Verification items for the finished model (mm, model axes). A direction names the side the tool comes from. Round coordinates to 2 decimals unless told otherwise and drop trailing zeros. Order: outer loops, then holes, each group sorted by start corner. A loop starts at its lowest first (then second) coordinate and runs counter-clockwise, first axis right, second up. Notation, with made-up numbers: (4.5, 28.25) -> (44.5, 28.25) arc R17 cw to (44.5, 37.25) -> close; hole circle Ø4 at (11.25, 34). An arc over 180 degrees is marked (long way). Put each result on its own line as item: value.
from build123d import *

# Parameters (mm, degrees)
ESQUISSE1_R             = 8
BOSS_EXTRU_1_DEPTH      = 5
ESQUISSE2_W             = 30
ESQUISSE2_H             = 12
BOSS_EXTRU_2_DEPTH      = 10.5
ESQUISSE4_W             = 30
ESQUISSE4_H             = 5
BOSS_EXTRU_3_DEPTH      = 45
ENL_V_START             = -10
ESQUISSE6_R             = 8
ENL_V_MAT_EXTRU_3_DEPTH = 10
ESQUISSE8_W             = 8
ESQUISSE8_H             = 8
ESQUISSE8_R             = 2.3
BOSS_EXTRU_4_DEPTH      = 8
ENL_V_MAT_EXTRU_4_DEPTH = 2
ENL_V_MAT_EXTRU_5_DEPTH = 50
ENL_V_MAT_EXTRU_6_DEPTH = 50
BOSS_EXTRU_5_DEPTH      = 10.5
BOSS_EXTRU_7_DEPTH      = 15


with BuildPart() as part:
    # Esquisse1 → Boss.-Extru.1 (new body)
    with BuildSketch(Plane.XY):
        Polygon((0, 0), (15, 0), (15, 45), (-15, 45), (-15, 0), align=None)
        with Locations((0, 28)):
            Circle(ESQUISSE1_R, mode=Mode.SUBTRACT)
    extrude(amount=-BOSS_EXTRU_1_DEPTH)

    # Esquisse2 → Boss.-Extru.2 (add)
    with BuildSketch(Plane(origin=(0, 0, -5), x_dir=(-1, 0, 0), z_dir=(0, 0, -1))):
        with Locations((0, 6)):
            Rectangle(ESQUISSE2_W, ESQUISSE2_H)
    extrude(amount=BOSS_EXTRU_2_DEPTH)

    # Esquisse4 → Boss.-Extru.3 (add)
    with BuildSketch(Plane.XZ):
        with Locations((0, -18)):
            Rectangle(ESQUISSE4_W, ESQUISSE4_H)
    extrude(amount=-BOSS_EXTRU_3_DEPTH)

    # Esquisse6 → Enlèv. mat.-Extru.3 (cut)
    with BuildSketch(Plane(origin=(0, 0, -20.5), x_dir=(-1, 0, 0), z_dir=(0, 0, -1)).offset(ENL_V_START)):
        with Locations(Location((0, 28, 0), (0, 0, 180))):
            Circle(ESQUISSE6_R)
    extrude(amount=ENL_V_MAT_EXTRU_3_DEPTH, mode=Mode.SUBTRACT)

    # Esquisse8 → Boss.-Extru.4 (add)
    # profile 1 of 4: a face of its own
    with BuildSketch(Plane.XZ):
        with Locations((-11, 4)):
            Rectangle(ESQUISSE8_W, ESQUISSE8_H)
        with Locations(Location((-11, 4, 0), (0, 0, 270))):
            Circle(ESQUISSE8_R, mode=Mode.SUBTRACT)
    # profile 2 of 4: a face of its own
    with BuildSketch(Plane.XZ):
        with Locations((11, 4)):
            Rectangle(ESQUISSE8_W, ESQUISSE8_H)
        with Locations(Location((11, 4, 0), (0, 0, 270))):
            Circle(ESQUISSE8_R, mode=Mode.SUBTRACT)
    # profile 3 of 4: a face of its own
    with BuildSketch(Plane.XZ):
        with Locations((-11, -24.5)):
            Rectangle(ESQUISSE8_W, ESQUISSE8_H)
        with Locations(Location((-11, -24.5, 0), (0, 0, 270))):
            Circle(ESQUISSE8_R, mode=Mode.SUBTRACT)
    # profile 4 of 4: a face of its own
    with BuildSketch(Plane.XZ):
        with Locations((11, -24.5)):
            Rectangle(ESQUISSE8_W, ESQUISSE8_H)
        with Locations(Location((11, -24.5, 0), (0, 0, 270))):
            Circle(ESQUISSE8_R, mode=Mode.SUBTRACT)
    extrude(amount=-BOSS_EXTRU_4_DEPTH)

    # Esquisse9 → Enlèv. mat.-Extru.4 (cut)
    with BuildSketch(Plane.XZ):
        Polygon((-15, 8), (-15, -28.5), (-7, -28.5), (-7, -20.5), (7, -20.5), (7, -28.5), (15, -28.5), (15, 8), (7, 8), (7, 0), (-7, 0), (-7, 8), align=None)
    extrude(amount=-ENL_V_MAT_EXTRU_4_DEPTH, mode=Mode.SUBTRACT)

    # Esquisse10 → Enlèv. mat.-Extru.5 (cut)
    with BuildSketch(Plane.ZY.offset(15)):
        with BuildLine():
            Line((-13.25, 2), (-7.25, 2))
            Line((-7.25, 2), (-7.25, 5.5))
            ThreePointArc((-7.25, 5.5), (-10.25, 8.5), (-13.25, 5.5))
            Line((-13.25, 5.5), (-13.25, 2))
        make_face()
    extrude(amount=-ENL_V_MAT_EXTRU_5_DEPTH, mode=Mode.SUBTRACT)

    # Esquisse11 → Enlèv. mat.-Extru.6 (cut)
    with BuildSketch(Plane.XY):
        Polygon((-9, 45), (-15, 45), (-15, 39), align=None)
        Polygon((15, 45), (9, 45), (15, 39), align=None)
    extrude(amount=-ENL_V_MAT_EXTRU_6_DEPTH, mode=Mode.SUBTRACT)

    # Esquisse12 → Boss.-Extru.5 (add)
    with BuildSketch(Plane(origin=(0, 0, -5), x_dir=(-1, 0, 0), z_dir=(0, 0, -1))):
        Polygon((0, 12), (15, 12), (15, 20), align=None)
    extrude(amount=BOSS_EXTRU_5_DEPTH)

    # Esquisse13 → Boss.-Extru.7 (add)
    with BuildSketch(Plane.XY.offset(-15.5)):
        Polygon((-15, 20), (-15, 39), (-10.757359313, 43.242640687), (-10.757359313, 17.084037873), align=None)
    extrude(amount=BOSS_EXTRU_7_DEPTH)


solid = part.part
Item 1: Section check C-C on z = -3. Record the boundary of the cut face in (x, y), then the cut area to 3 significant figures.
Check sheet entries:
outline: (-15, 2) -> (15, 2) -> (15, 39) -> (9, 45) -> (-9, 45) -> (-15, 39) -> close; hole circle Ø16 at (0, 28)
area: 1,050 mm^2
Item 2: Section check A-A on y = 28. Record the boundary of the cut face in (x, z).
Check sheet entries:
outline: (-15, -20.5) -> (-8, -20.5) -> (-8, -15.5) -> (-10.76, -15.5) -> (-10.76, -5) -> (-8, -5) -> (-8, 0) -> (-15, 0) -> close; (8, -20.5) -> (15, -20.5) -> (15, -15.5) -> (8, -15.5) -> close; (8, -5) -> (15, -5) -> (15, 0) -> (8, 0) -> close
Item 3: Tool access check on faces 1 (the flat face through (-5.454, 14.909, -10.176)), 2 (the flat face through (-13, 8, 2)), 3 (the flat face through (-13, 8, -26)). Record the directions out of +Z, -Z, +X, -X, +Y, -Y that give a thin tool (end or side, any length) a straight path to the whole face; none if there is none.
Check sheet entries:
face 1: +X, +Y
face 2: +Z, +X, -X, +Y
face 3: -Z, +X, -X, +Y
Item 4: Section check D-D on z = 4. Record the boundary of the cut face in (x, y).
Check sheet entries:
outline: (-15, 2) -> (-13.3, 2) -> (-13.3, 8) -> (-15, 8) -> close; (-8.7, 2) -> (-7, 2) -> (-7, 8) -> (-8.7, 8) -> close; (7, 2) -> (8.7, 2) -> (8.7, 8) -> (7, 8) -> close; (13.3, 2) -> (15, 2) -> (15, 8) -> (13.3, 8) -> close
Item 5: Section check B-B on x = 11. Record the boundary of the cut face in (y, z), then the cut area to 3 significant figures.
Check sheet entries:
outline: (2, -28.5) -> (8, -28.5) -> (8, -26.8) -> (2, -26.8) -> close; (2, -22.2) -> (8, -22.2) -> (8, -20.5) -> (43, -20.5) -> (43, -15.5) -> (12, -15.5) -> (12, -5) -> (43, -5) -> (43, 0) -> (8, 0) -> (8, 1.7) -> (2, 1.7) -> (2, -7.25) -> (5.5, -7.25) arc R3 cw to (5.5, -13.25) -> (2, -13.25) -> close; (2, 6.3) -> (8, 6.3) -> (8, 8) -> (2, 8) -> close
area: 521 mm^2
Item 6: Release check for a two-part mould opening along X. For faces 4 (the cylindrical face through (-8.72, 4.96, 4.3)), 5 (the flat face through (0, 2, -1)), 6 (the flat face through (-15, 20, -10)) record: +X half, -X half, draft (parallel to the pull), parting line (faces both ways), or undercut.
Check sheet entries:
face 4: undercut
face 5: draft
face 6: -X half
Item 7: Gauge pin test, flat ends, axial feed: pin 1 Ø1.5 at (x, z) = (-6.5, -8.5) entering from +Y; pin 2 Ø9 at (x, y) = (3, 25.5) entering from -Z; pin 3 Ø2.5 at (x, z) = (-12.5, 3) entering from +Y. Record the tip position at first contact, or that the pin passes through.
Check sheet entries:
pin 1: stops at y = 15.87
pin 2: stops at z = -20.5
pin 3: stops at y = 8
Item 8: Material ranges on L1, parallel to X at y = 6.1, z = -24.5; L2, parallel to Z at x = -9.75, y = 43; L3, parallel to X at y = 5, z = -24 (3 decimals), recorded low to high. Write a range as [from, to].
Check sheet entries:
L1: x = [-15, -13.3], [-8.7, -7], [7, 8.7], [13.3, 15]
L2: z = [-20.5, -15.5], [-5, 0]
L3: x = [-15, -13.245], [-8.755, -7], [7, 8.755], [13.245, 15]
